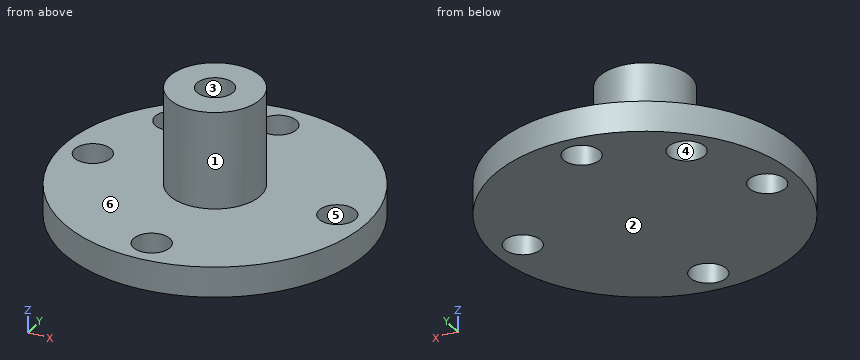
Autodesk Inventor part; units mm, degrees
ref_plane "YZ Plane" through (0, 0, 0) normal (1, 0, 0) x (0, 1, 0)
ref_plane "XZ Plane" through (0, 0, 0) normal (0, 1, 0) x (-1, 0, 0)
ref_plane "XY Plane" through (0, 0, 0) normal (0, 0, 1) x (1, 0, 0)
sketch "Sketch1" plane through (0, 0, 0) normal (0, 0, 1) x (1, 0, 0)
  circle A0 centre (0, 0) radius 25
  dimension "d0" = 50
extrude "Extrusion1" add sketch "Sketch1" along normal blind 5
sketch "Sketch2" plane through (0, 0, 5) normal (0, 0, 1) x (1, 0, 0)
  circle A0 centre (0, 20) radius 3
  circle A1 centre (20, 0) radius 3
  circle A2 centre (-20, 0) radius 3
  circle A3 centre (0, -20) radius 3
  dimension "d4" = 6
  dimension "d5" = 6
  dimension "d6" = 6
  dimension "d7" = 6
hole "Hole1" at (-20, 0, 5) at (0, 20, 5) at (20, 0, 5) at (0, -20, 5) direction (0, 0, -1) diameter 6 end through all
thread "Thread1"
thread "Thread2"
thread "Thread3"
thread "Thread4"
pattern_circular "Circular Pattern1" count 2 over 45 about axis through (0, 0, 0) along (0, 0, 1) of "Hole1"
sketch "Sketch4" plane through (0, 0, 5) normal (0, 0, 1) x (1, 0, 0)
  circle A0 centre (14.1421, 14.1421) radius 3
  circle A1 centre (14.1421, 14.1421) radius 3
  circle A2 centre (14.1421, -14.1421) radius 3
  circle A3 centre (14.1421, -14.1421) radius 3
  circle A4 centre (-14.1421, -14.1421) radius 3
  circle A5 centre (-14.1421, -14.1421) radius 3
  point P0 (0, 0)
extrude "Extrusion2" add sketch "Sketch4" against normal blind 5
sketch "Sketch5" plane through (0, 0, 5) normal (0, 0, 1) x (1, 0, 0)
  circle A0 centre (-14.1421, 14.1421) radius 3
  circle A1 centre (20, 0) radius 3
  circle A2 centre (-20, 0) radius 3
  circle A3 centre (0, 20) radius 3
  circle A4 centre (0, -20) radius 3
  circle A5 centre (0, 0) radius 25
  circle A6 centre (0, 0) radius 7.5
  circle A7 centre (0, 0) radius 3
  dimension "d29" = 15
  dimension "d30" = 6
extrude "Extrusion3" add sketch "Sketch5" along normal blind 16 contours A6
properties part number "Base"
The model under review builds one solid part; all positions refer to its coordinate system, in mm. Face numbers are marked on the shaded views. A direction names the side the tool comes from. Give positions to 0.01 mm unless a question says otherwise; leave off trailing zeros. Loops run counter-clockwise (first coordinate to the right, second up) from the corner with the lowest first, then second, coordinate; pieces in that order, holes last. Notation, with made-up numbers: (57.25, 89) -> (98.25, 89) arc R28 ccw to (98.25, 109) -> close; hole circle Ø6 at (40, 45). An arc over 180 degrees is marked (long way). Write each question's results on one line, items separated by ' | '.
1) For line 1 along Y through (x, z) = (0, 1.7); line 2 along Y through (x, z) = (0, 15); line 3 along Z through (x, y) = (14, -12), list the stretches that pass through material, from the lowest coordinate up. Write a range as from..to.
Conclusion:
line 1: y = -25..-23, -17..17, 23..25 | line 2: y = -7.5..-3, 3..7.5 | line 3: z = 0..5
2) Draft analysis for pull direction Y (two halves, no side actions). For the marked faces 1, 2, 3 and 4, state which applies: pulls with the +Y half, pulls with the -Y half, needs draft (parallel to the pull), parting line crosses it, or undercut.
Conclusion:
face 1: parting line crosses it | face 2: needs draft | face 3: undercut | face 4: undercut
3) Take a section at D-D, the plane z = 7.5. Give the boundary of the cut face in (x, y), plus the area to 3 significant figures.
Conclusion:
outline: circle Ø15 at (0, 0); hole circle Ø6 at (0, 0) | area: 148 mm^2
4) Tool access review of the marked faces 5 and 6: name each direction out of +Z, -Z, +X, -X, +Y, -Y from which nothing blocks a thin tool from reaching the whole face with its end or side.
Conclusion:
face 5: +Z, -Z | face 6: +Z
5) Insertion check: pin 1 Ø5 at (x, y) = (-1, 1.5) entering from +Z; pin 2 Ø12 at (x, z) = (-2.5, 13) entering from +Y; pin 3 Ø1.5 at (x, y) = (2, 14) entering from +Z; pin 4 Ø4 at (x, z) = (8, 10) entering from +Y. Each pin has a flat end and moves straight along its axis. Give the tip position at first contact, or say it passes through.
Conclusion:
pin 1: stops at z = 21 | pin 2: stops at y = 7.5 | pin 3: stops at z = 5 | pin 4: stops at y = 4.5
6) Take a section at A-A, the plane y = 20. Give the boundary of the cut face in (x, z).
Conclusion:
outline: (-15, 0) -> (-3, 0) -> (-3, 5) -> (-15, 5) -> close; (3, 0) -> (15, 0) -> (15, 5) -> (3, 5) -> close
7) Take a section at B-B, the plane y = 0. Give the boundary of the cut face in (x, z).
Conclusion:
outline: (-25, 0) -> (-23, 0) -> (-23, 5) -> (-25, 5) -> close; (-17, 0) -> (17, 0) -> (17, 5) -> (7.5, 5) -> (7.5, 21) -> (3, 21) -> (3, 5) -> (-3, 5) -> (-3, 21) -> (-7.5, 21) -> (-7.5, 5) -> (-17, 5) -> close; (23, 0) -> (25, 0) -> (25, 5) -> (23, 5) -> close
